from build123d import *

# Parameters (mm, degrees)
F0_W      = 159.258
F0_H      = 25.4
F1_DEPTH  = 50.8
F3_DEPTH  = 50.801
F4_R      = 0.762
F5_R      = 0.508
F7_W      = 145.288
F7_H      = 44.45
F8_DEPTH  = 22.226
F9_W      = 3.175
F9_H      = 44.45
F10_DEPTH = 22.225
F11_R     = 3.175


with BuildPart() as f1:
    # F0 (on Front) → F1 (new body)
    with BuildSketch(Plane.XZ):
        with Locations((0, -12.7)):
            Rectangle(F0_W, F0_H)
    extrude(amount=-F1_DEPTH)

    # F2 (on face) → F3 (cut, through all)
    with BuildSketch(Plane.XZ):
        Polygon((-77.851, -7.112), (-79.629, -7.112), (-79.629, -25.4), (-75.819, -25.4), (-75.819, -5.588), (-77.851, -5.588), align=None)
        Polygon((77.851, -5.588), (75.819, -5.588), (75.819, -25.4), (79.629, -25.4), (79.629, -7.112), (77.851, -7.112), align=None)
    extrude(amount=-F3_DEPTH, mode=Mode.SUBTRACT)

    # F4
    f4_edges = [f1.edges().sort_by_distance(p)[0] for p in [
        (-79.629, 25.4, -7.112),
        (-77.851, 25.4, -7.112),
        (77.851, 25.4, -7.112),
        (79.629, 25.4, -7.112),
    ]]
    fillet(f4_edges, radius=F4_R)

    # F5
    f5_edges = [f1.edges().sort_by_distance(p)[0] for p in [
        (-77.851, 25.4, -5.588),
        (-75.819, 25.4, -5.588),
        (77.851, 25.4, -5.588),
        (75.819, 25.4, -5.588),
    ]]
    fillet(f5_edges, radius=F5_R)

    # F7 (on offset) → F8 (cut, through all)
    with BuildSketch(Plane(origin=(0, 0, -22.225), x_dir=(1, 0, 0), z_dir=(0, 0, -1))):
        with Locations((0, -25.4)):
            Rectangle(F7_W, F7_H)
    extrude(amount=-F8_DEPTH, mode=Mode.SUBTRACT)

    # F9 (on face) → F10 (join, through all)
    with BuildSketch(Plane.XY.offset(-22.225)):
        with Locations((-23.4315, 25.4)):
            Rectangle(F9_W, F9_H)
        with Locations((23.4315, 25.4)):
            Rectangle(F9_W, F9_H)
    extrude(amount=F10_DEPTH)

    # F11
    f11_edges = [f1.edges().sort_by_distance(p)[0] for p in [
        (-25.019, 25.4, -22.225),
        (-48.8315, 47.625, -22.225),
        (-72.644, 25.4, -22.225),
        (-48.8315, 3.175, -22.225),
        (21.844, 25.4, -22.225),
        (0, 47.625, -22.225),
        (-21.844, 25.4, -22.225),
        (0, 3.175, -22.225),
        (72.644, 25.4, -22.225),
        (48.8315, 47.625, -22.225),
        (25.019, 25.4, -22.225),
        (48.8315, 3.175, -22.225),
    ]]
    fillet(f11_edges, radius=F11_R)


solid = f1.part
The listing builds one solid part. Answer for the finished solid, in the listing's coordinates (mm). A direction names the side the tool comes from. Give positions to 0.01 mm unless a question says otherwise; leave off trailing zeros. Order: outer loops, then holes, each group sorted by start corner. A loop starts at its lowest first (then second) coordinate and runs counter-clockwise, first axis right, second up. Notation, with made-up numbers: (40, 29.25) -> (55, 29.25) arc R11 cw to (55, 50.25) -> close; hole circle Ø9 at (-24, 71.25). An arc over 180 degrees is marked (long way). Put each result on its own line as item: value.
Item 1: Straight lines are drawn through the part: line 1 (X direction, y = 18, z = -8.75); line 2 (X direction, y = 11, z = -2.75); line 3 (Y direction, x = -63, z = -18.5) (3 decimals). For each, find the intervals that lie inside material, in ascending order.
Established:
line 1: x = -75.82 to -72.64, -25.02 to -21.84, 21.84 to 25.02, 72.64 to 75.82
line 2: x = -79.63 to -72.64, -25.02 to -21.84, 21.84 to 25.02, 72.64 to 79.63
line 3: y = 0 to 3.175, 47.625 to 50.8
Item 2: A cutting plane is placed at B-B on z = -15.5. Give the vertices of the cut face in (x, y) (3 decimals).
Established:
outline: (-75.819, 0) -> (75.819, 0) -> (75.819, 50.8) -> (-75.819, 50.8) -> close; hole (-72.644, 3.175) -> (-25.019, 3.175) -> (-25.019, 47.625) -> (-72.644, 47.625) -> close; hole (-21.844, 3.175) -> (21.844, 3.175) -> (21.844, 47.625) -> (-21.844, 47.625) -> close; hole (25.019, 3.175) -> (72.644, 3.175) -> (72.644, 47.625) -> (25.019, 47.625) -> close
Item 3: For faces 5 (the face through (-21.844, 25, -10)), 6 (the face through (0, 3, 0)), determine the directions among +Z, -Z, +X, -X, +Y, -Y from which every point of the face is accessible in a straight line to the end or side of a thin tool.
Established:
face 5: +Z
face 6: +Z, +X, -X, +Y, -Y
Item 4: A cutting plane is placed at A-A on x = 54. Give the vertices of the cut face in (y, z) (3 decimals), plus the area to 3 significant figures.
Established:
outline: (0, -25.4) -> (50.8, -25.4) -> (50.8, 0) -> (47.625, 0) -> (47.625, -19.05) arc R3.175 cw to (44.45, -22.225) -> (6.35, -22.225) arc R3.175 cw to (3.175, -19.05) -> (3.175, 0) -> (0, 0) -> close
area: 307 mm^2
Item 5: Given P1, Ø1.5, axis at x = 40, y = 16.5, coming from the +Z side (3 decimals); P2, Ø0.5, axis at x = -77, y = 20, coming from the -Z side; P3, Ø9.5, axis at y = 32, z = -13.5, coming from the +X side, each flat-ended and moving along its own axis, determine where each tip first touches the part or whether it passes through.
Established:
P1: stops at z = -22.225
P2: stops at z = -5.59
P3: stops at x = 75.82
Item 6: A cutting plane is placed at C-C on z = -1.5. Give the vertices of the cut face in (x, y) (3 decimals), plus the area to 3 significant figures.
Established:
outline: (-79.629, 0) -> (79.629, 0) -> (79.629, 50.8) -> (-79.629, 50.8) -> close; hole (-72.644, 3.175) -> (-25.019, 3.175) -> (-25.019, 47.625) -> (-72.644, 47.625) -> close; hole (-21.844, 3.175) -> (21.844, 3.175) -> (21.844, 47.625) -> (-21.844, 47.625) -> close; hole (25.019, 3.175) -> (72.644, 3.175) -> (72.644, 47.625) -> (25.019, 47.625) -> close
area: 1,910 mm^2
Item 7: For a pull along Y with two mould halves and no side action, classify faces 1 (the face through (0.31, 46.72, -21.27)), 2 (the face through (-1, 50.8, -13)), 3 (the face through (79.629, 25, -3)), 4 (the face through (-1, 0, -13)) as released by +Y, released by -Y, zero draft, split by the parting line, or undercut.
Established:
face 1: undercut
face 2: released by +Y
face 3: zero draft
face 4: released by -Y
